Source: CAD feature listing. Evaluate the final solid. Frame: model axes, mm. A direction names the side the tool comes from. Coordinates: 2 decimals unless noted, no trailing zeros. Order: outer loops, then holes, each group sorted by start corner. A loop starts at its lowest first (then second) coordinate and runs counter-clockwise, first axis right, second up.
```python
from build123d import *

# Parameters (mm, degrees)
F1_DEPTH = 1056
F3_DEPTH = 10
F5_DEPTH = 10


with BuildPart() as f1:
    # F0 (on Right) → F1 (new body)
    with BuildSketch(Plane.YZ):
        Polygon((0, 75.7), (0, 0), (38, 0), (38, 91.440115), align=None)
    extrude(amount=-F1_DEPTH)

    # F2 (on face) → F3 (join)
    with BuildSketch(Plane.YZ):
        Polygon((25, 86.055339), (25, 0), (38, 0), (38, 91.440115), align=None)
    extrude(amount=F3_DEPTH)

    # F4 (on face) → F5 (join)
    with BuildSketch(Plane(origin=(-1056, 0, 0), x_dir=(0, -1, 0), z_dir=(-1, 0, 0))):
        Polygon((-38, 0), (-25, 0), (-25, 86.055339), (-38, 91.440115), align=None)
    extrude(amount=F5_DEPTH)


solid = f1.part
```
1. Section query A-A on y = 31. Return loops of the section in (x, z).
Findings:
outline: (-1066, 0) - (10, 0) - (10, 88.54) - (-1066, 88.54) - close
2. Access query for faces 1 (the face through (-1056, 12, 44)), 2 (the face through (-520, 19, 0)), 3 (the face through (0, 12, 44)). Directions: +Z, -Z, +X, -X, +Y, -Y. A direction counts if a zero-diameter tool reaches every point of the face in a straight line with its end or side. Return the directions, or none.
Findings:
face 1: +Z, -Z, -X, -Y
face 2: -Z, +X, -X, +Y, -Y
face 3: +Z, -Z, +X, -Y
3. Section query B-B on x = -210.5. Return loops of the section in (y, z).
Findings:
outline: (0, 0) - (38, 0) - (38, 91.44) - (0, 75.7) - close
4. Ray query, line 1 (X direction, y = 9.5, z = 79.5); line 2 (Y direction, x = -836.5, z = 86); line 3 (Z direction, x = -953.5, y = 24.5). Return the intervals inside material, ascending.
Findings:
line 1: x = -1056 to 0
line 2: y = 24.87 to 38
line 3: z = 0 to 85.85
5. Pin query (flat end, axial travel): P1, Ø2, axis at y = 8.5, z = 45.5, coming from the +X side; P2, Ø11, axis at x = 2.5, z = 56.5, coming from the -Y side; P3, Ø8, axis at y = 9.5, z = 27.5, coming from the -X side; P4, Ø3, axis at x = -1063, z = 40, coming from the -Y side. Return the tip coordinate at first contact, or that it passes through.
Findings:
P1: stops at x = 0
P2: stops at y = 0
P3: stops at x = -1056
P4: stops at y = 25
